Design review of the part built by this model. Coordinates are the model's own, in mm. A direction names the side the tool comes from. Coordinates: 2 decimals unless noted, no trailing zeros. Write each loop counter-clockwise with the first axis right and the second up, starting at its lowest first coordinate (ties: lowest second). Pieces come first, ordered by that corner, then holes. Notation, with made-up numbers: (-17.5, 29) - (12.5, 29) arc R21 ccw to (12.5, 51) - close; hole circle Ø2 at (42.5, 32.5). An arc over 180 degrees is marked (long way). Use a Markdown table: item, result.
from build123d import *

# Parameters (mm, degrees)
F0_W     = 50
F0_H     = 40
F0_R     = 3
F0_W_2   = 8.5
F0_H_2   = 4
F0_R_2   = 3.425
F0_W_3   = 4.5
F0_H_3   = 9.5
F1_DEPTH = 2
F2_R     = 1


with BuildPart() as f1:
    # F0 (on Top) → F1 (new body)
    with BuildSketch(Plane.XY):
        with Locations((11.034863, 15.014281)):
            Rectangle(F0_W, F0_H)
        with Locations((10.034863, 1.014281)):
            Circle(F0_R, mode=Mode.SUBTRACT)
        with Locations((21.534863, 1.214281)):
            Rectangle(F0_W_2, F0_H_2, mode=Mode.SUBTRACT)
        with Locations((-0.465137, 29.514281)):
            Circle(F0_R_2, mode=Mode.SUBTRACT)
        with Locations((28.784863, 27.514281)):
            Rectangle(F0_W_3, F0_H_3, mode=Mode.SUBTRACT)
    extrude(amount=F1_DEPTH)

    # F2
    f2_edges = [f1.edges().sort_by_distance(p)[0] for p in [
        (31.034863, 27.514281, 2),
        (28.784863, 22.764281, 2),
        (26.534863, 27.514281, 2),
        (28.784863, 32.264281, 2),
        (17.284863, 1.214281, 2),
        (21.534863, -0.785719, 2),
        (25.784863, 1.214281, 2),
        (21.534863, 3.214281, 2),
        (7.034863, 1.014281, 2),
        (-3.890137, 29.514281, 2),
        (11.034863, 35.014281, 2),
        (-13.965137, 15.014281, 2),
        (36.034863, 15.014281, 2),
        (11.034863, -4.985719, 2),
    ]]
    fillet(f2_edges, radius=F2_R)


solid = f1.part
(1) Draft analysis for pull direction Y (two halves, no side actions). For faces 1 (the flat face through (11, 15, 2)), 2 (the cylindrical face through (21.6, 3.5, 1.7)), 3 (the cylindrical face through (11.38, 34.73, 1.7)), state which applies: +Y half, -Y half, draft (parallel to the pull), parting line (faces both ways), or undercut.
Determined:
| item | result |
|---|---|
| face 1 | draft |
| face 2 | undercut |
| face 3 | +Y half |
(2) For pin 1 (3.5 mm diameter, centred on x = 10.03, y = 1.01, fed in from +Z), flat-tipped, find the tip position at first contact; note if it passes through.
Determined:
| item | result |
|---|---|
| pin 1 | through |
(3) Machinability: for faces 4 (the flat face through (11, 15, 0)), 5 (the cylindrical face through (28.83, 32.55, 1.7)), 6 (the flat face through (31.035, 27.4, 0.5)), which of the approach directions +Z, -Z, +X, -X, +Y, -Y give a long, thin tool a straight path to every point of the face, cutting with its end or side? Answer none if there is none.
Determined:
| item | result |
|---|---|
| face 4 | -Z, +X, -X, +Y, -Y |
| face 5 | +Z |
| face 6 | +Z, -Z |
(4) Take a section at B-B on y = 24. Write out the cut boundary in (x, z).
Determined:
| item | result |
|---|---|
| outline | (-13.97, 0) - (26.53, 0) - (26.53, 1) arc R1 ccw to (25.53, 2) - (-12.97, 2) arc R1 ccw to (-13.97, 1) - close; (31.03, 0) - (36.03, 0) - (36.03, 1) arc R1 ccw to (35.03, 2) - (32.03, 2) arc R1 ccw to (31.03, 1) - close |
(5) Take a section at C-C on z = 1.45. Write out the cut boundary in (x, y), and give its area (3 significant figures).
Determined:
| item | result |
|---|---|
| outline | (-13.86, -4.88) - (35.93, -4.88) - (35.93, 34.91) - (-13.86, 34.91) - close; hole circle Ø7.06 at (-0.47, 29.51); hole circle Ø6.21 at (10.03, 1.01); hole (17.18, -0.89) - (25.89, -0.89) - (25.89, 3.32) - (17.18, 3.32) - close; hole (26.43, 22.66) - (31.14, 22.66) - (31.14, 32.37) - (26.43, 32.37) - close |
| area | 1,830 mm2 |
(6) For L1, parallel to X at y = 23, z = 0.75; L2, parallel to Y at x = 24.5, z = 0.1; L3, parallel to Y at x = 28.5, z = 0.95, list the stretches that pass through material, from the lowest coordinate up. Write a range as from..to.
Determined:
| item | result |
|---|---|
| L1 | -13.97..26.53, 31.03..36.03 |
| L2 | -4.99..-0.79, 3.21..35.01 |
| L3 | -4.99..22.76, 32.26..35.01 |
(7) Take a section at D-D on y = 0. State how many separate pieces and enclosed holes the cut face has, and give its area (3 significant figures).
Determined:
| item | result |
|---|---|
| separate pieces | 3 |
| enclosed holes | 0 |
| area | 70.4 mm2 |
(8) Take a section at A-A on x = 29. Write out the cut boundary in (y, z), and give its area (3 significant figures).
Determined:
| item | result |
|---|---|
| outline | (-4.99, 0) - (22.76, 0) - (22.76, 1) arc R1 ccw to (21.76, 2) - (-3.99, 2) arc R1 ccw to (-4.99, 1) - close; (32.26, 0) - (35.01, 0) - (35.01, 1) arc R1 ccw to (34.01, 2) - (33.26, 2) arc R1 ccw to (32.26, 1) - close |
| area | 60.1 mm2 |
